```python
from build123d import *

# Parameters (mm, degrees)
F0_W     = 150
F0_H     = 350
F1_DEPTH = 25
F2_R     = 50
F4_D     = 50


with BuildPart() as f1:
    # F0 (on Front) → F1 (new body)
    with BuildSketch(Plane.XZ):
        with Locations((94.000003, 175)):
            Rectangle(F0_W, F0_H)
    extrude(amount=F1_DEPTH)

    # F2
    f2_edges = [f1.edges().sort_by_distance(p)[0] for p in [
        (19.000003, -12.5, 350),
        (169.000003, -12.5, 350),
    ]]
    fillet(f2_edges, radius=F2_R)

    # F4 (through all)
    with Locations(Plane.XZ.offset(25)):
        with Locations((94.000003, 250)):
            Hole(F4_D / 2)


solid = f1.part
```
Check sheet for the modelled part. Datum: model origin and axes. Units: mm. Coordinates: 2 decimals unless noted, no trailing zeros. Write each loop counter-clockwise with the first axis right and the second up, starting at its lowest first coordinate (ties: lowest second). Pieces come first, ordered by that corner, then holes. Notation, with made-up numbers: (78, 63) -> (86, 63) arc R30 cw to (86, 89) -> close; hole circle Ø6 at (30.25, -25.75). An arc over 180 degrees is marked (long way). Use a Markdown table: item, result.
1. Sectioned sample at B-B (z = 250). Enter the section's corners in (x, y), plus the area to 3 significant figures.
Reported:
| item | result |
|---|---|
| outline | (19, -25) -> (69, -25) -> (69, 0) -> (19, 0) -> close; (119, -25) -> (169, -25) -> (169, 0) -> (119, 0) -> close |
| area | 2,500 mm2 |
2. Release check for a two-part mould opening along X. For faces 1 (the cylindrical face through (154.742, -12.675, 334.964)), 2 (the flat face through (93, -12, 0)), 3 (the cylindrical face through (97.255, -12.325, 274.787)), 4 (the flat face through (19, -12, 148)) record: pulls with the +X half, pulls with the -X half, needs draft (parallel to the pull), parting line crosses it, or undercut.
Reported:
| item | result |
|---|---|
| face 1 | pulls with the +X half |
| face 2 | needs draft |
| face 3 | undercut |
| face 4 | pulls with the -X half |
3. Go/stop test with a flat-tipped pin: pin 1 Ø2 at (x, y) = (46, -19.5) entering from -Z. Record where the tip stops, or that it passes through.
Reported:
| item | result |
|---|---|
| pin 1 | stops at z = 0 |
4. Sectioned sample at D-D (x = 147.5). Enter the section's corners in (y, z).
Reported:
| item | result |
|---|---|
| outline | (-25, 0) -> (0, 0) -> (0, 341.08) -> (-25, 341.08) -> close |
5. Sectioned sample at C-C (x = 89). Enter the section's corners in (y, z), plus the area to 3 significant figures.
Reported:
| item | result |
|---|---|
| outline | (-25, 0) -> (0, 0) -> (0, 225.51) -> (-25, 225.51) -> close; (-25, 274.49) -> (0, 274.49) -> (0, 350) -> (-25, 350) -> close |
| area | 7,530 mm2 |
6. Scan lines: line 1 along Z through (x, y) = (103.5, -17.75); line 2 along Z through (x, y) = (148.5, -9); line 3 along Z through (x, y) = (132, -12.25). Record each from-to range of solid material in increasing order.
Reported:
| item | result |
|---|---|
| line 1 | z = 0 to 226.88, 273.12 to 350 |
| line 2 | z = 0 to 340.37 |
| line 3 | z = 0 to 348.28 |
7. Sectioned sample at A-A (y = -21.5). Enter the section's corners in (x, z).
Reported:
| item | result |
|---|---|
| outline | (19, 0) -> (169, 0) -> (169, 300) arc R50 ccw to (119, 350) -> (69, 350) arc R50 ccw to (19, 300) -> close; hole circle Ø50 at (94, 250) |
